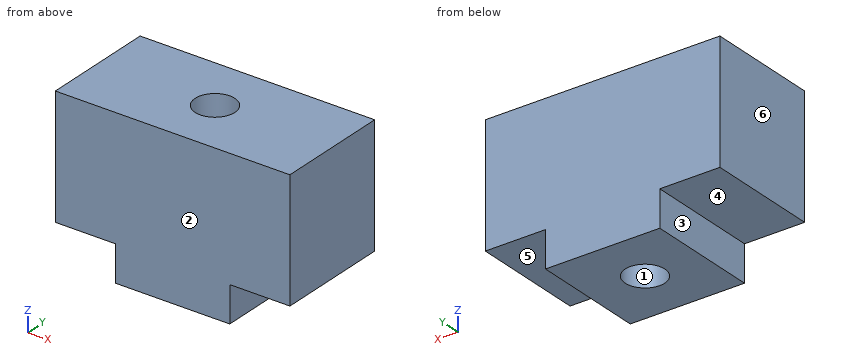
```python
from build123d import *

# Parameters (mm, degrees)
F1_DEPTH = 9.5
F2_R     = 1.65
F3_DEPTH = 13.001


with BuildPart() as f1:
    # F0 (on Front) → F1 (new body)
    with BuildSketch(Plane.XZ):
        Polygon((9.75, 10), (0, 10), (-9.75, 10), (-9.75, 0), (-4.75, 0), (-4.75, -3), (0, -3), (4.75, -3), (4.75, 0), (9.75, 0), align=None)
    extrude(amount=F1_DEPTH)

    # F2 (on face) → F3 (cut, through all)
    with BuildSketch(Plane.XY.offset(10)):
        with Locations((0, -4.75)):
            Circle(F2_R)
    extrude(amount=-F3_DEPTH, mode=Mode.SUBTRACT)


solid = f1.part
```
For this review, take the finished solid that the model builds, in its own axes (mm). Face numbers are marked on the shaded views. A direction names the side the tool comes from. Round coordinates to 2 decimals unless told otherwise and drop trailing zeros. Write each loop counter-clockwise with the first axis right and the second up, starting at its lowest first coordinate (ties: lowest second). Pieces come first, ordered by that corner, then holes. Notation, with made-up numbers: (69.5, 27) -> (118.5, 27) arc R21 ccw to (118.5, 42) -> close; hole circle Ø7 at (-36, 18). An arc over 180 degrees is marked (long way). Use one line per item in the form item = value.
1) Take a section at C-C, the plane y = -4.75. Write out the cut boundary in (x, z).
Found:
outline = (-9.75, 0) -> (-4.75, 0) -> (-4.75, -3) -> (-1.65, -3) -> (-1.65, 10) -> (-9.75, 10) -> close; (1.65, -3) -> (4.75, -3) -> (4.75, 0) -> (9.75, 0) -> (9.75, 10) -> (1.65, 10) -> close
2) Take a section at A-A, the plane x = 0. Write out the cut boundary in (y, z).
Found:
outline = (-9.5, -3) -> (-6.4, -3) -> (-6.4, 10) -> (-9.5, 10) -> close; (-3.1, -3) -> (0, -3) -> (0, 10) -> (-3.1, 10) -> close
3) Clearance check with flat-ended pins moving along their axes: pin 1 (4 mm diameter, centred on x = -8.5, y = -5, fed in from -Z); pin 2 (2.5 mm diameter, centred on x = 0, y = -4.75, fed in from -Z) (3 decimals); pin 3 (0.9 mm diameter, centred on y = -6.5, z = -1.5, fed in from +X). State where each tip first meets the part, or that it passes through.
Found:
pin_1 = 0
pin_2 = through
pin_3 = 4.75
4) Tool access review of the marked faces 4, 5 and 6: name each direction out of +Z, -Z, +X, -X, +Y, -Y from which nothing blocks a thin tool from reaching the whole face with its end or side.
Found:
face_4 = -Z, -X, +Y, -Y
face_5 = -Z, +X, +Y, -Y
face_6 = +Z, -Z, -X, +Y, -Y
5) Mouldability with a two-part tool opening along X and no side actions: class the marked faces 1, 2 and 3 as +X half, -X half, draft (parallel to the pull), parting line (faces both ways), or undercut.
Found:
face_1 = undercut
face_2 = draft
face_3 = -X half
6) Take a section at D-D, the plane x = 7. Write out the cut boundary in (y, z), and give its area (3 significant figures).
Found:
outline = (-9.5, 0) -> (0, 0) -> (0, 10) -> (-9.5, 10) -> close
area = 95.0 mm2
7) To check wall thickness, follow L1, parallel to Y at x = 0, z = 2.25; L2, parallel to Z at x = 9, y = -7; L3, parallel to Y at x = -0.5, z = 3.25. State the ranges of each line that lie inside material, in increasing order. Write a range as from..to.
Found:
L1 = -9.5..-6.4, -3.1..0
L2 = 0..10
L3 = -9.5..-6.32, -3.18..0
8) Take a section at B-B, the plane z = -0.5. Write out the cut boundary in (x, y).
Found:
outline = (-4.75, -9.5) -> (4.75, -9.5) -> (4.75, 0) -> (-4.75, 0) -> close; hole circle Ø3.3 at (0, -4.75)
